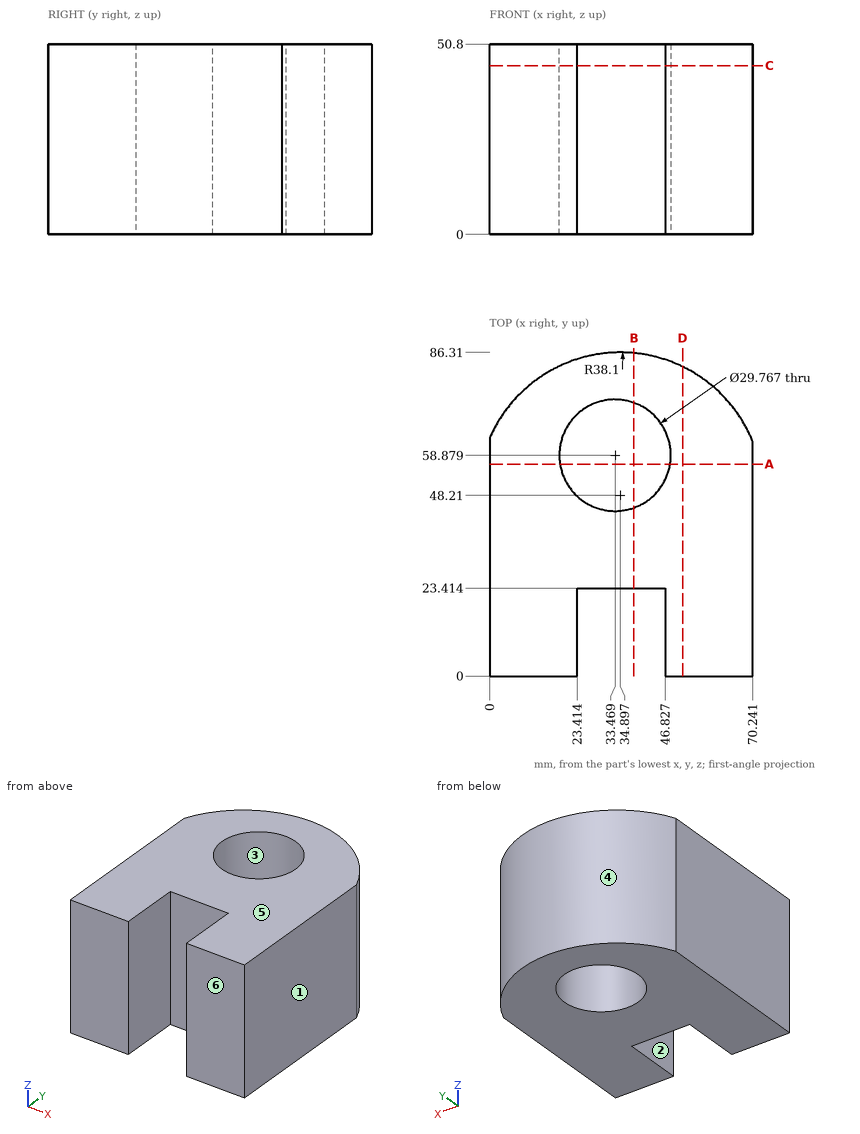
Drawing for the job (mm, zero at the part's lowest x, y, z). A direction names the side the tool comes from. Give positions to 0.01 mm unless a question says otherwise; leave off trailing zeros. Order: outer loops, then holes, each group sorted by start corner. A loop starts at its lowest first (then second) coordinate and runs counter-clockwise, first axis right, second up. Notation, with made-up numbers: (67, 16.5) - (73, 16.5) arc R21 cw to (73, 35.5) - close; hole circle Ø3 at (27.5, 10.5). An arc over 180 degrees is marked (long way). Write item = value, one per line. Start each with the question number.
1. Probe line 1 along X through (y, z) = (19, 39); line 2 along X through (y, z) = (46, 13.5) (1 decimal); line 3 along Y through (x, z) = (44, 46) (1 decimal). List the from-to ranges inside material, lowest first.
2. Cut at A-A, the plane y = 56.5. List the corners of the cut face in (x, z), and give its area (3 significant figures).
3. Cut at C-C, the plane z = 45. List the corners of the cut face in (x, y).
4. Two-plate mould, pull along Y, no slides. Class the marked faces 3, 4, 5 and 6: pulls with the +Y half, pulls with the -Y half, needs draft (parallel to the pull), parting line crosses it, or undercut.
5. Drop flat-ended pins along their axis: P1, Ø8, axis at x = 18.5, z = 13.5, coming from the +Y side; P2, Ø5, axis at x = 8, y = 32.5, coming from the -Z side; P3, Ø7, axis at x = 37.5, z = 28.5, coming from the -Y side; P4, Ø10, axis at x = 10.5, z = 22, coming from the +Y side. Give the stop position or say it passes through.
6. Cut at D-D, the plane x = 51.5. List the corners of the cut face in (y, z), and give its area (3 significant figures).
7. Cut at B-B, the plane x = 38.5. List the corners of the cut face in (y, z), and give its area (3 significant figures).
8. Which spindle directions (+Z, -Z, +X, -X, +Y, -Y) get a long thin tool onto all of the face, cutting with end or side? Do the marked faces 1 and 2. Say none if no direction does.
Taken from the geometry:
q1.line_1 = 0 to 23.41, 46.83 to 70.24
q1.line_2 = 0 to 26, 40.9 to 70.2
q1.line_3 = 23.4 to 48.4, 69.4 to 85.2
q2.outline = (0, 0) - (18.78, 0) - (18.78, 50.8) - (0, 50.8) - close; (48.16, 0) - (70.24, 0) - (70.24, 50.8) - (48.16, 50.8) - close
q2.area = 2,080 mm²
q3.outline = (0, 0) - (23.41, 0) - (23.41, 23.41) - (46.83, 23.41) - (46.83, 0) - (70.24, 0) - (70.24, 62.44) arc R38.1 ccw to (0, 63.5) - close; hole circle Ø29.77 at (33.47, 58.88)
q4.face_3 = undercut
q4.face_4 = pulls with the +Y half
q4.face_5 = needs draft
q4.face_6 = pulls with the -Y half
q5.P1 = 84.24
q5.P2 = 0
q5.P3 = 23.41
q5.P4 = 81
q6.outline = (0, 0) - (82.5, 0) - (82.5, 50.8) - (0, 50.8) - close
q6.area = 4,190 mm²
q7.outline = (23.41, 0) - (44.87, 0) - (44.87, 50.8) - (23.41, 50.8) - close; (72.89, 0) - (86.14, 0) - (86.14, 50.8) - (72.89, 50.8) - close
q7.area = 1,760 mm²
q8.face_1 = +Z, -Z, +X, +Y, -Y
q8.face_2 = +Z, -Z, -Y
